Answer from the drawing. Dimensions are ordinates in mm from the lowest x, y and z of the part. Give positions to 0.01 mm unless a question says otherwise; leave off trailing zeros. Order: outer loops, then holes, each group sorted by start corner. A loop starts at its lowest first (then second) coordinate and runs counter-clockwise, first axis right, second up. Notation, with made-up numbers: (-24.5, -17.75) - (13.5, -17.75) arc R8 cw to (13.5, -13.75) - close; hole circle Ø11 at (5, -1.75). An arc over 180 degrees is marked (long way). Write each question's results on one line, items separated by ' | '.
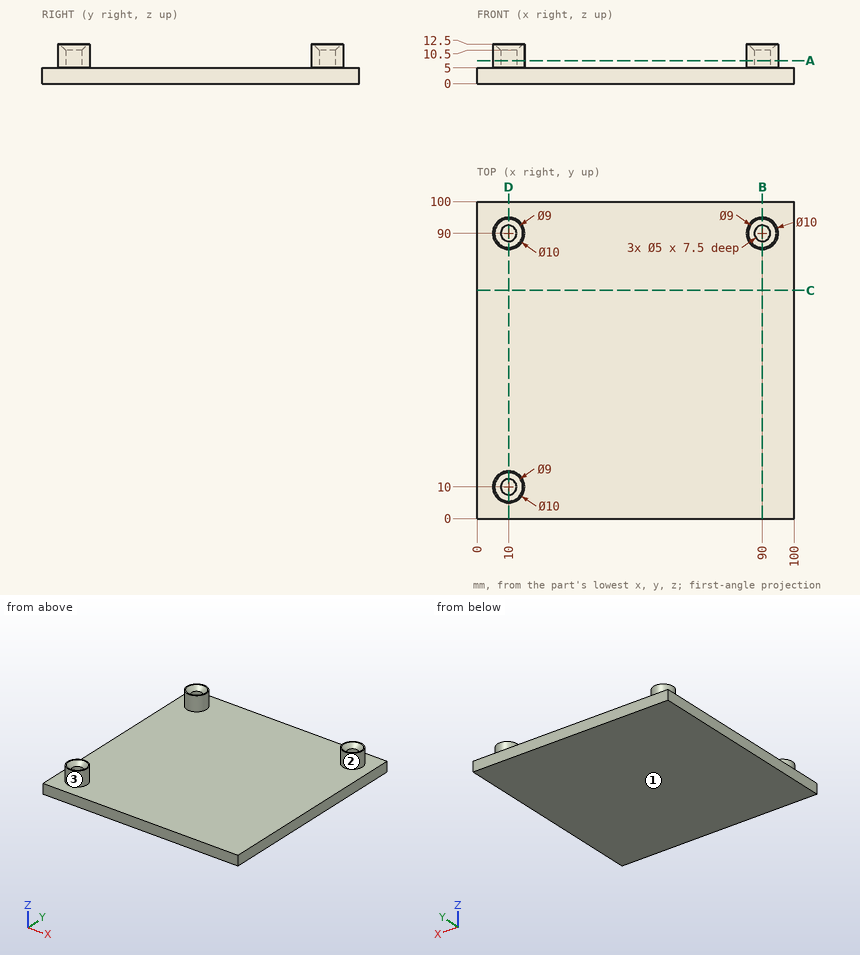
1. Straight lines are drawn through the part: line 1 (Y direction, x = 10, z = 7.95); line 2 (Z direction, x = 35, y = 14); line 3 (Y direction, x = 90, z = 6.75). For each, find the intervals that lie inside material, in ascending order. Write a range as [from, to].
Answer list:
line 1: [5, 7.5], [12.5, 15], [85, 87.5], [92.5, 95] | line 2: [0, 5] | line 3: [85, 87.5], [92.5, 95]
2. A cutting plane is placed at A-A, the plane z = 7.25. Write down the section's boundary in (x, y), then the cut area to 3 significant figures.
Answer list:
outline: circle Ø10 at (10, 10); circle Ø10 at (10, 90); circle Ø10 at (90, 90); hole circle Ø5 at (10, 10); hole circle Ø5 at (10, 90); hole circle Ø5 at (90, 90) | area: 177 mm^2
3. A cutting plane is placed at C-C, the plane y = 72. Write down the section's boundary in (x, z).
Answer list:
outline: (0, 0) - (100, 0) - (100, 5) - (0, 5) - close
4. Determine the mould class of the marked faces 1, 2 and 3 for opening direction X: +X half, -X half, draft (parallel to the pull), parting line (faces both ways), or undercut.
Answer list:
face 1: draft | face 2: undercut | face 3: parting line
5. A cutting plane is placed at D-D, the plane x = 10. Write down the section's boundary in (y, z).
Answer list:
outline: (0, 0) - (100, 0) - (100, 5) - (95, 5) - (95, 12.5) - (94.5, 12.5) - (92.5, 10.5) - (92.5, 5) - (87.5, 5) - (87.5, 10.5) - (85.5, 12.5) - (85, 12.5) - (85, 5) - (15, 5) - (15, 12.5) - (14.5, 12.5) - (12.5, 10.5) - (12.5, 5) - (7.5, 5) - (7.5, 10.5) - (5.5, 12.5) - (5, 12.5) - (5, 5) - (0, 5) - close
6. A cutting plane is placed at B-B, the plane x = 90. Write down the section's boundary in (y, z), then the cut area to 4 significant figures.
Answer list:
outline: (0, 0) - (100, 0) - (100, 5) - (95, 5) - (95, 12.5) - (94.5, 12.5) - (92.5, 10.5) - (92.5, 5) - (87.5, 5) - (87.5, 10.5) - (85.5, 12.5) - (85, 12.5) - (85, 5) - (0, 5) - close | area: 533.5 mm^2
7. Given P1, Ø1, axis at x = 44.5, y = 21.5, coming from the +Z side; P2, Ø5.5, axis at x = 9, y = 90, coming from the +Z side; P3, Ø1.5, axis at x = 70, z = 6.5, coming from the +Y side; P4, Ø8, axis at x = 10, y = 90, coming from the +Z side, each flat-ended and moving along its own axis, determine where each tip first touches the part or whether it passes through.
Answer list:
P1: z = 5 | P2: z = 11.75 | P3: through | P4: z = 12
